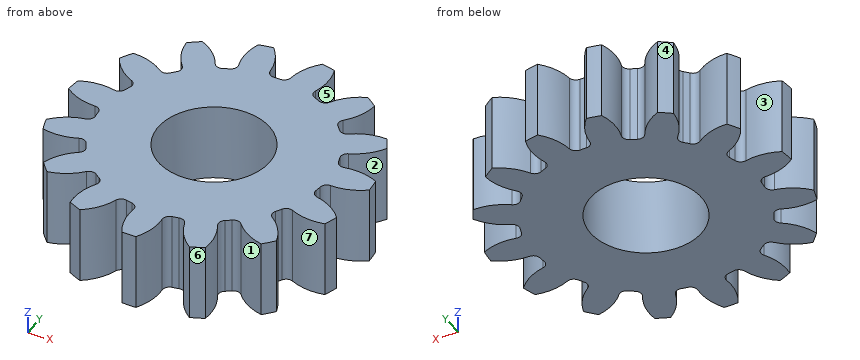
from build123d import *

# Parameters (mm, degrees)
SKETCH3_R         = 21.59
GEARBODY_DEPTH    = 11
TOOTHCUT_DEPTH    = 12
CIRPATTERN1_COUNT = 15
BOREDIA_R         = 7.874
BORE_DEPTH        = 12700


with BuildPart() as part:
    # Sketch3 → gearBody (new body)
    with BuildSketch(Plane.XY):
        Circle(SKETCH3_R)
    extrude(amount=GEARBODY_DEPTH)

    # Sketch2 → toothCut (cut, through all)
    with BuildSketch(Plane.XY):
        with BuildLine():
            ThreePointArc((15.783846764, -2.304552616), (15.843293638, -1.852249483), (15.889781974, -1.39843136))
            ThreePointArc((15.889781974, -1.39843136), (16.213055843, -0.751556907), (16.890861518, -0.499501321))
            ThreePointArc((16.890861518, -0.499501321), (20.504912911, 0.340315353), (23.283949955, 2.798691365))
            ThreePointArc((23.283949955, 2.798691365), (23.292901215, -2.723187818), (22.010467945, -8.09409042))
            ThreePointArc((22.010467945, -8.09409042), (19.873444675, -5.060974685), (16.550574786, -3.410158156))
            ThreePointArc((16.550574786, -3.410158156), (15.949189176, -3.008551507), (15.783846764, -2.304552616))
        make_face()
    toothcut = extrude(amount=TOOTHCUT_DEPTH, mode=Mode.SUBTRACT)

    # CirPattern1: toothCut ×15 about axis
    cirpattern1_axis = Axis((0, 0, 0), (0, 0, 1))
    for i in range(1, CIRPATTERN1_COUNT):
        add(toothcut.rotate(cirpattern1_axis, i * 360 / CIRPATTERN1_COUNT), mode=Mode.SUBTRACT)

    # boreDia → bore (cut, symmetric)
    with BuildSketch(Plane.XY):
        Circle(BOREDIA_R)
    extrude(amount=BORE_DEPTH, both=True, mode=Mode.SUBTRACT)


solid = part.part
Input: part model. Units: mm. Frame: model coordinates. Face numbers are marked on the shaded views. A direction names the side the tool comes from. Round coordinates to 2 decimals unless told otherwise and drop trailing zeros. Write each loop counter-clockwise with the first axis right and the second up, starting at its lowest first coordinate (ties: lowest second). Pieces come first, ordered by that corner, then holes.
1) Cut plane A-A (y = -10.5). Return the cut outline in (x, z), then the cut area to 3 significant figures.
2) Reachability of the marked faces 1, 2 and 3 from +Z, -Z, +X, -X, +Y, -Y: full face, straight path, thin tool, end or side. Return the list, or none.
3) Draft query along Y for the marked faces 4, 5, 6 and 7. Return one class per face: pulls with the +Y half, pulls with the -Y half, needs draft (parallel to the pull), parting line crosses it, or undercut.
4) Contact query for flat-ended pins moving along their axis: P1, Ø1.5, axis at y = 2, z = 9.5, coming from the +X side; P2, Ø5, axis at x = 12.5, z = 4.5, coming from the -Y side; P3, Ø1, axis at y = 11.5, z = 2.5, coming from the -X side. Output: stop coordinate, or through.
5) Ray query, L1, parallel to Y at x = 19, z = 4.5; L2, parallel to Y at x = 0, z = 2.5; L3, parallel to X at y = 15.5, z = 5. Return the intervals inside material, ascending.
Geometry says:
1. outline: (-15.1, 0) - (14.51, 0) - (14.51, 11) - (-15.1, 11) - close
1. area: 326 mm2
2. face 1: +Z, -Z, -Y
2. face 2: +Z, -Z, +X
2. face 3: +Z, -Z
3. face 4: pulls with the +Y half
3. face 5: undercut
3. face 6: pulls with the -Y half
3. face 7: undercut
4. P1: stops at x = 21.55
4. P2: stops at y = -15.32
4. P3: stops at x = -18.58
5. L1: y = -8.02 to -4.41, -0.24 to 3.72, 9.21 to 10.25
5. L2: y = -21.59 to -7.87, 7.87 to 15.95
5. L3: x = -13.03 to -8.4, -5.3 to 5.64, 8.9 to 13.48
